```python
from build123d import *

# Parameters (mm, degrees)
F0_W     = 22
F0_H     = 2450
F1_DEPTH = 45
F3_D     = 3
F3_DEPTH = 22
F5_D     = 18


with BuildPart() as f1:
    # F0 (on Front) → F1 (new body)
    with BuildSketch(Plane.XZ):
        Rectangle(F0_W, F0_H)
    extrude(amount=F1_DEPTH)

    # F3
    with Locations(Plane.XZ.offset(45)):
        with Locations((0, 1195), (0, 770), (0, -505), (0, 345), (0, -930), (0, -80)):
            Hole(F3_D / 2, depth=F3_DEPTH)

    # F5 (through all)
    with Locations(Plane.YZ.offset(11)):
        with Locations((-22.5, 1195), (-22.5, 770), (-22.5, 345), (-22.5, -80), (-22.5, -505), (-22.5, -930)):
            Hole(F5_D / 2)


solid = f1.part
```
The listing builds one solid part. Answer for the finished solid, in the listing's coordinates (mm). Give positions to 0.01 mm unless a question says otherwise; leave off trailing zeros. Order: outer loops, then holes, each group sorted by start corner. A loop starts at its lowest first (then second) coordinate and runs counter-clockwise, first axis right, second up. Notation, with made-up numbers: (62, -10.75) - (115, -10.75) arc R18 cw to (115, 1.25) - close; hole circle Ø2 at (67, 63.25). An arc over 180 degrees is marked (long way). Use one line per item in the form item = value. Start each with the question number.
(1) A cutting plane is placed at A-A, the plane y = -22.5. Write down the section's boundary in (x, z), then the cut area to 3 significant figures.
(2) A flat-ended cylindrical pin translates along its axis: pin 1 Ø2.5 at (x, z) = (0, -80) entering from -Y. Find the tip coordinate at first contact, or state that the pin passes through.
(3) Consider line 1 (X direction, y = -39.5, z = 770); line 2 (Y direction, x = 0.25, z = -930). Determine where each line is inside the solid, lowest interval first. Write a range as from..to.
Ans:
q1.outline = (-11, -1225) - (11, -1225) - (11, -939) - (-11, -939) - close; (-11, -921) - (11, -921) - (11, -514) - (-11, -514) - close; (-11, -496) - (11, -496) - (11, -89) - (-11, -89) - close; (-11, -71) - (11, -71) - (11, 336) - (-11, 336) - close; (-11, 354) - (11, 354) - (11, 761) - (-11, 761) - close; (-11, 779) - (11, 779) - (11, 1186) - (-11, 1186) - close; (-11, 1204) - (11, 1204) - (11, 1225) - (-11, 1225) - close
q1.area = 51,500 mm^2
q2.pin_1 = -13.59
q3.line_1 = -11..-1.5, 1.5..11
q3.line_2 = -13.5..0
